from build123d import *

# Parameters (mm, degrees)
F0_W     = 50.8
F0_H     = 50.8
F1_DEPTH = 6.35
F2_W     = 50.8
F2_H     = 25.4
F3_DEPTH = 12.7
F4_W     = 12.7
F4_H     = 25.4
F5_DEPTH = 12.7
F7_D     = 6.35


with BuildPart() as f1:
    # F0 (on Top) → F1 (new body, symmetric)
    with BuildSketch(Plane.XY):
        with Locations((6.228447, 33.990965)):
            Rectangle(F0_W, F0_H)
    extrude(amount=F1_DEPTH, both=True)

    # F2 (on face) → F3 (join, symmetric)
    with BuildSketch(Plane.XY.offset(6.35)):
        with Locations((6.228447, 21.290965)):
            Rectangle(F2_W, F2_H)
    extrude(amount=F3_DEPTH, both=True)

    # F4 (on face) → F5 (join, symmetric)
    with BuildSketch(Plane.XY.offset(6.35)):
        with Locations((-12.821553, 46.690965)):
            Rectangle(F4_W, F4_H)
    extrude(amount=F5_DEPTH, both=True)

    # F7 (through all)
    with Locations(Plane.YZ.offset(-6.471553)):
        with Locations((46.690965, 12.7)):
            Hole(F7_D / 2)


solid = f1.part
Design review of the part built by this model. Coordinates are the model's own, in mm. A direction names the side the tool comes from. Coordinates: 2 decimals unless noted, no trailing zeros. Order: outer loops, then holes, each group sorted by start corner. A loop starts at its lowest first (then second) coordinate and runs counter-clockwise, first axis right, second up. Notation, with made-up numbers: (43, -16.5) - (70, -16.5) arc R6 ccw to (70, -9.5) - close; hole circle Ø2 at (40.5, 68). An arc over 180 degrees is marked (long way). Put each result on its own line as item: value.
1) Wall thickness on L1, parallel to Z at x = 19, y = 55; L2, parallel to Y at x = 7, z = 11; L3, parallel to Y at x = -13, z = 14: over which ranges is each line inside the solid? List them lowest first. Write a range as from..to.
Response values:
L1: z = -6.35..6.35
L2: y = 8.59..33.99
L3: y = 8.59..43.79, 49.59..59.39
2) Take a section at C-C, the plane y = 36.5. Give the boundary of the cut face in (x, z), and give its area (3 significant figures).
Response values:
outline: (-19.17, -6.35) - (31.63, -6.35) - (31.63, 6.35) - (-6.47, 6.35) - (-6.47, 19.05) - (-19.17, 19.05) - close
area: 806 mm²
3) The part is to be moulded in two halves that separate along Z. For faces 1 (the face through (-12.91, 43.76, 11.48)), 2 (the face through (31.628, 28, 4)), 3 (the face through (6, 34, -6.35)), 4 (the face through (0, 23, 19.05)), say which applies: released by +Z, released by -Z, zero draft, split by the parting line, or undercut.
Response values:
face 1: undercut
face 2: zero draft
face 3: released by -Z
face 4: released by +Z
4) Tool access review of faces 5 (the face through (0, 59.391, 1)), 6 (the face through (12, 33.991, 13)): name each direction out of +Z, -Z, +X, -X, +Y, -Y from which nothing blocks a thin tool from reaching the whole face with its end or side.
Response values:
face 5: +Z, -Z, +X, -X, +Y
face 6: +Z, +X, +Y
5) Take a section at A-A, the plane z = 12.7. Give the boundary of the cut face in (x, y).
Response values:
outline: (-19.17, 8.59) - (31.63, 8.59) - (31.63, 33.99) - (-6.47, 33.99) - (-6.47, 43.52) - (-19.17, 43.52) - close; (-19.17, 49.87) - (-6.47, 49.87) - (-6.47, 59.39) - (-19.17, 59.39) - close
6) Insertion check: P1, Ø1.5, axis at x = -4.5, y = 41.5, coming from the +Z side; P2, Ø1, axis at y = 42.5, z = 16, coming from the +X side; P3, Ø5, axis at y = 46.69, z = 12.7, coming from the -X side; P4, Ø14, axis at x = 22, z = 13, coming from the +Y side. Each pin has a flat end and moves straight along its axis. Give the tip position at first contact, or say it passes through.
Response values:
P1: stops at z = 6.35
P2: stops at x = -6.47
P3: passes through
P4: stops at y = 59.39
7) Take a section at B-B, the plane x = -13.5. Give the boundary of the cut face in (y, z) (3 decimals).
Response values:
outline: (8.591, -6.35) - (59.391, -6.35) - (59.391, 19.05) - (8.591, 19.05) - close; hole circle Ø6.35 at (46.691, 12.7)
8) Take a section at D-D, the plane x = 3. Give the boundary of the cut face in (y, z), and give its area (3 significant figures).
Response values:
outline: (8.59, -6.35) - (59.39, -6.35) - (59.39, 6.35) - (33.99, 6.35) - (33.99, 19.05) - (8.59, 19.05) - close
area: 968 mm²
